Design review of the part built by this model. Coordinates are the model's own, in mm. Face numbers are marked on the shaded views. Give positions to 0.01 mm unless a question says otherwise; leave off trailing zeros. Order: outer loops, then holes, each group sorted by start corner. A loop starts at its lowest first (then second) coordinate and runs counter-clockwise, first axis right, second up. Notation, with made-up numbers: (-37.5, 11.5) -> (3.5, 11.5) arc R21 ccw to (3.5, 29.5) -> close; hole circle Ø10 at (36.5, 62). An arc over 180 degrees is marked (long way). Return JSON: item names as keys, results as strings.
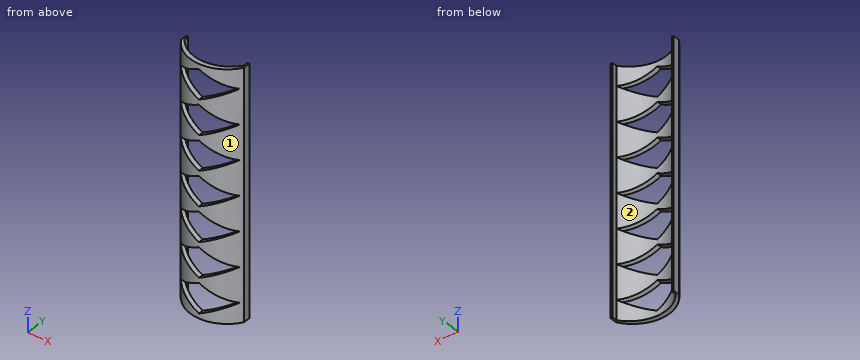
```python
from build123d import *

# Parameters (mm, degrees)
F1_DEPTH = 250
F3_DEPTH = 250
F5_DEPTH = 37.501


# Not quite as in the source:
# - a feature names something its author has since deleted; it is built from what else it names


with BuildPart() as f1:
    # F0 (on Top) → F1 (new body)
    with BuildSketch(Plane.XY):
        with BuildLine():
            Line((-32, -12.551214796), (-32, -19.551214796))
            ThreePointArc((-32, -19.551214796), (0, -37.5), (32, -19.551214796))
            Line((32, -19.551214796), (32, -12.551214796))
            Line((32, -12.551214796), (0, -12.551214796))
            Line((0, -12.551214796), (-32, -12.551214796))
        make_face()
    extrude(amount=F1_DEPTH)

    # F2 (on face) → F3 (cut)
    with BuildSketch(Plane(origin=(0, 0, 0), x_dir=(1, 0, 0), z_dir=(0, 0, -1))):
        with BuildLine():
            Line((-30, 12.551214796), (30, 12.551214796))
            Line((30, 12.551214796), (30, 17.551214796))
            ThreePointArc((30, 17.551214796), (0, 32.551214796), (-30, 17.551214796))
            Line((-30, 17.551214796), (-30, 12.551214796))
        make_face()
    extrude(amount=-F3_DEPTH, mode=Mode.SUBTRACT)

    # F4 (on Front) → F5 (cut, through all)
    with BuildSketch(Plane.XZ):
        Polygon((-30, 20), (0, 5), (30, 20), (0, 35), align=None)
        Polygon((0, 40), (30, 55), (0, 70), (-30, 55), align=None)
        Polygon((0, 110), (30, 125), (0, 140), (-30, 125), align=None)
        Polygon((0, 145), (30, 160), (0, 175), (-30, 160), align=None)
        Polygon((0, 180), (30, 195), (0, 210), (-30, 195), align=None)
        Polygon((0, 215), (30, 230), (0, 245), (-30, 230), align=None)
        Polygon((0, 75), (30, 90), (0, 105), (-30, 90), align=None)
    extrude(amount=F5_DEPTH, mode=Mode.SUBTRACT)


solid = f1.part
```
Item 1: For pin 1 (3 mm diameter, centred on x = 6.5, z = 184.5, fed in from -Y); pin 2 (4 mm diameter, centred on x = 15.5, z = 103.5, fed in from -Y); pin 3 (6 mm diameter, centred on y = -33, z = 178.5, fed in from +X); pin 4 (6 mm diameter, centred on x = -23, y = -19, fed in from -Z), all flat-tipped, find the tip position at first contact; note any pin that passes through.
Result set:
{"pin 1": "stops at y = -37", "pin 2": "stops at y = -34.99", "pin 3": "stops at x = 22.5", "pin 4": "passes through"}
Item 2: Mouldability with a two-part tool opening along X and no side actions: class the marked faces 1 and 2 as released by +X, released by -X, zero draft, split by the parting line, or undercut.
Result set:
{"face 1": "split by the parting line", "face 2": "undercut"}
Item 3: Add section A-A (x = 19). Give the number of separate pieces and of enclosed holes in the cut face, plus the area to 3 significant figures.
Result set:
{"separate pieces": "8", "enclosed holes": "0", "area": "856 mm^2"}
Item 4: Add section C-C (y = -15). Give the boundary of the cut face in (x, z).
Result set:
{"outline": "(-32, 0) -> (-30, 0) -> (-30, 250) -> (-32, 250) -> close; (30, 0) -> (32, 0) -> (32, 250) -> (30, 250) -> close"}
Item 5: Add section B-B (z = 155). Give the boundary of the cut face in (x, y).
Result set:
{"outline": "(-32, -19.55) arc R37.5 ccw to (-20, -31.72) -> (-20, -26.77) arc R37.5 cw to (-30, -17.55) -> (-30, -12.55) -> (-32, -12.55) -> close; (20, -31.72) arc R37.5 ccw to (32, -19.55) -> (32, -12.55) -> (30, -12.55) -> (30, -17.55) arc R37.5 cw to (20, -26.77) -> close"}
Item 6: Wall thickness on L1, parallel to X at y = -17.25, z = 127; L2, parallel to X at y = -20.25, z = 111; L3, parallel to Y at x = -29, z = 88: over which ranges is each line inside the solid? List them lowest first. Write a range as [from, to].
Result set:
{"L1": "x = [-32, -30], [30, 32]", "L2": "x = [-31.56, -27.77], [27.77, 31.56]", "L3": "y = [-23.77, -18.83]"}
